```python
from build123d import *

# Parameters (mm, degrees)
SKETCH1_R           = 1.6
BOSS_EXTRUDE1_DEPTH = 1.6


with BuildPart() as part:
    # Sketch1 → Boss-Extrude1 (new body)
    with BuildSketch(Plane(origin=(0, 0, 0), x_dir=(1, 0, 0), z_dir=(0, 1, 0))):
        Polygon((65.6, 0), (65.6, 2.6), (68.4, 5.4), (68.4, 37.9), (65.6, 40.7), (65.6, 52), (64.3, 53.3), (0, 53.3), (0, 0), align=None)
        with Locations(Location((65.9, 7.6, 0), (0, 0, 270))):
            Circle(SKETCH1_R, mode=Mode.SUBTRACT)
        with Locations(Location((65.9, 35.55, 0), (0, 0, 270))):
            Circle(SKETCH1_R, mode=Mode.SUBTRACT)
        with Locations(Location((15.4, 50.6, 0), (0, 0, 270))):
            Circle(SKETCH1_R, mode=Mode.SUBTRACT)
    extrude(amount=BOSS_EXTRUDE1_DEPTH)


solid = part.part
```
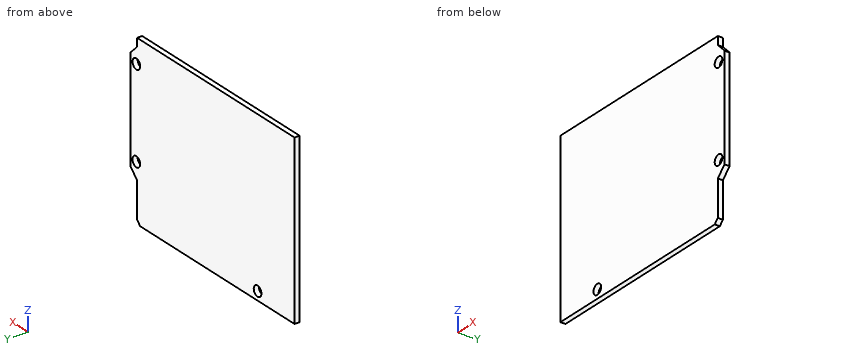
Source: CAD feature listing. Evaluate the final solid. Frame: model axes, mm. Coordinates: 2 decimals unless noted, no trailing zeros. Write each loop counter-clockwise with the first axis right and the second up, starting at its lowest first coordinate (ties: lowest second). Pieces come first, ordered by that corner, then holes. Notation, with made-up numbers: (47, 40.25) -> (73, 40.25) arc R22 cw to (73, 50.25) -> close; hole circle Ø7 at (44.5, 9). An arc over 180 degrees is marked (long way). Return JSON: item names as keys, results as strings. Group by question number.
1) Contact query for a flat-ended pin moving along its axis: P1, Ø0.8, axis at y = 1, z = -1, coming from the +X side. Output: stop coordinate, or through.
2) Ray query, line 1 along X through (y, z) = (1, -50.6); line 2 along Z through (x, y) = (65.9, 0.5); line 3 along X through (y, z) = (0.4, -7.6). Return the intervals inside material, ascending.
3) Section query A-A, the plane x = 15.4. Return loops of the section in (y, z), plus the area to 3 significant figures.
4) Section query C-C, the plane y = 1.3. Return loops of the section in (x, z), plus the area to 3 significant figures.
5) Section query B-B, the plane z = -50.6. Return loops of the section in (x, y), plus the area to 3 significant figures.
From the geometry:
{
 "1": {"P1": "x = 65.6"},
 "2": {"line 1": "0 to 13.8, 17 to 65.6", "line 2": "-40.4 to -37.15, -33.95 to -9.2, -6 to -2.9", "line 3": "0 to 64.3, 67.5 to 68.4"},
 "3": {"outline": "(0, -53.3) -> (1.6, -53.3) -> (1.6, -52.2) -> (0, -52.2) -> close; (0, -49) -> (1.6, -49) -> (1.6, 0) -> (0, 0) -> close", "area": "80.2 mm²"},
 "4": {"outline": "(0, -53.3) -> (64.3, -53.3) -> (65.6, -52) -> (65.6, -40.7) -> (68.4, -37.9) -> (68.4, -5.4) -> (65.6, -2.6) -> (65.6, 0) -> (0, 0) -> close; hole circle Ø3.2 at (15.4, -50.6); hole circle Ø3.2 at (65.9, -35.55); hole circle Ø3.2 at (65.9, -7.6)", "area": "3,570 mm²"},
 "5": {"outline": "(0, 0) -> (13.8, 0) -> (13.8, 1.6) -> (0, 1.6) -> close; (17, 0) -> (65.6, 0) -> (65.6, 1.6) -> (17, 1.6) -> close", "area": "99.8 mm²"}
}
